The model under review builds one solid part; all positions refer to its coordinate system, in mm. A direction names the side the tool comes from. Round coordinates to 2 decimals unless told otherwise and drop trailing zeros. Loops run counter-clockwise (first coordinate to the right, second up) from the corner with the lowest first, then second, coordinate; pieces in that order, holes last. Notation, with made-up numbers: (-29.5, 60) -> (0.5, 60) arc R36 cw to (0.5, 99) -> close; hole circle Ø2 at (9.25, -5). An arc over 180 degrees is marked (long way). Use a Markdown table: item, result. Add a question column.
1) Consider section B-B on x = 3.25. State how many separate pieces and enclosed holes the cut face has, plus the area to 3 significant figures.
2) For faces 1 (the flat face through (3.11, -0.98, -6.9)), 2 (the cylindrical face through (5.314, -0.083, 2.217)), 3 (the flat face through (3.106, 2.602, -6.468)), list the 3-axis set-ups (+Z, -Z, +X, -X, +Y, -Y) from which the entire face can be reached by the end or side of a thin tool; tool diameter is ignored.
3) Consider section A-A on y = 0. Give the boundary of the cut face in (x, z).
4) Insertion check: pin 1 (3.5 mm diameter, centred on y = 0, z = 4.42, fed in from +X); pin 2 (3 mm diameter, centred on x = 1, z = 7, fed in from +Y). Each pin has a flat end and moves straight along its axis. Give the tip position at first contact, or say it passes through.
5) Wall thickness on probe 1 along Z at (x, y) = (0.75, 0.25); probe 2 along Y at (x, z) = (3.5, 7.75); probe 3 along Z at (x, y) = (3.75, -0.5): over which ranges is each line inside the solid? List them lowest first.
6) Mouldability with a two-part tool opening along Y and no side actions: class faces 4 (the flat face through (3.11, -6.46, 2.6)), 5 (the cylindrical face through (3.106, 4.579, -4.564)), 6 (the flat face through (0, 0, 0)) as released by +Y, released by -Y, zero draft, split by the parting line, or undercut.
from build123d import *

# Parameters (mm, degrees)
BOSS_EXTRUDE1_DEPTH = 6.3
SKETCH2_R           = 1.1
CUT_EXTRUDE1_DEPTH  = 7.3000001
SKETCH3_R           = 2.2
CUT_EXTRUDE2_DEPTH  = 2


with BuildPart() as part:
    # Sketch1 → Boss-Extrude1 (new body)
    with BuildSketch(Plane(origin=(0, 0, 0), x_dir=(0, 0, -1), z_dir=(1, 0, 0))):
        with BuildLine():
            Line((-0.909343603, 6.400728022), (-1.05, 7.390786494))
            add(Edge.make_bspline(
                [(-0.410905417, 9.290786494), (-0.761226832, 8.915917898), (-1.03420339, 8.440297341), (-1.05, 7.390786494)],
                knots=[0, 0, 0, 0, 1, 1, 1, 1], degree=3))
            Line((-0.410905417, 9.290786494), (0.410905417, 9.290786494))
            add(Edge.make_bspline(
                [(0.410905417, 9.290786494), (0.761226832, 8.915917898), (1.03420339, 8.440297341), (1.05, 7.390786494)],
                knots=[0, 0, 0, 0, 1, 1, 1, 1], degree=3))
            Line((1.05, 7.390786494), (0.909343603, 6.400728022))
            ThreePointArc((0.909343603, 6.400728022), (1.673265127, 6.244710467), (2.41284935, 5.997864871))
            Line((2.41284935, 5.997864871), (2.786066573, 6.925608858))
            add(Edge.make_bspline(
                [(4.289538717, 8.251509833), (3.798717175, 8.102024814), (3.324502262, 7.826613608), (2.786066573, 6.925608858)],
                knots=[0, 0, 0, 0, 1, 1, 1, 1], degree=3))
            Line((4.289538717, 8.251509833), (5.001247777, 7.840604417))
            add(Edge.make_bspline(
                [(5.001247777, 7.840604417), (5.117200723, 7.340797982), (5.115795079, 6.792410217), (4.604719921, 5.875608858)],
                knots=[0, 0, 0, 0, 1, 1, 1, 1], degree=3))
            Line((4.604719921, 5.875608858), (3.987878672, 5.088521268))
            ThreePointArc((3.987878672, 5.088521268), (4.57144534, 4.57144534), (5.088521268, 3.987878672))
            Line((5.088521268, 3.987878672), (5.875608858, 4.604719921))
            add(Edge.make_bspline(
                [(7.840604417, 5.001247777), (7.340797982, 5.117200723), (6.792410217, 5.115795079), (5.875608858, 4.604719921)],
                knots=[0, 0, 0, 0, 1, 1, 1, 1], degree=3))
            Line((7.840604417, 5.001247777), (8.251509833, 4.289538717))
            add(Edge.make_bspline(
                [(8.251509833, 4.289538717), (8.102024814, 3.798717175), (7.826613608, 3.324502262), (6.925608858, 2.786066573)],
                knots=[0, 0, 0, 0, 1, 1, 1, 1], degree=3))
            Line((6.925608858, 2.786066573), (5.997864871, 2.41284935))
            ThreePointArc((5.997864871, 2.41284935), (6.244710467, 1.673265127), (6.400728022, 0.909343603))
            Line((6.400728022, 0.909343603), (7.390786494, 1.05))
            add(Edge.make_bspline(
                [(9.290786494, 0.410905417), (8.915917898, 0.761226832), (8.440297341, 1.03420339), (7.390786494, 1.05)],
                knots=[0, 0, 0, 0, 1, 1, 1, 1], degree=3))
            Line((9.290786494, 0.410905417), (9.290786494, -0.410905417))
            add(Edge.make_bspline(
                [(9.290786494, -0.410905417), (8.915917898, -0.761226832), (8.440297341, -1.03420339), (7.390786494, -1.05)],
                knots=[0, 0, 0, 0, 1, 1, 1, 1], degree=3))
            Line((7.390786494, -1.05), (6.400728022, -0.909343603))
            ThreePointArc((6.400728022, -0.909343603), (6.244710467, -1.673265127), (5.997864871, -2.41284935))
            Line((5.997864871, -2.41284935), (6.925608858, -2.786066573))
            add(Edge.make_bspline(
                [(8.251509833, -4.289538717), (8.102024814, -3.798717175), (7.826613608, -3.324502262), (6.925608858, -2.786066573)],
                knots=[0, 0, 0, 0, 1, 1, 1, 1], degree=3))
            Line((8.251509833, -4.289538717), (7.840604417, -5.001247777))
            add(Edge.make_bspline(
                [(7.840604417, -5.001247777), (7.340797982, -5.117200723), (6.792410217, -5.115795079), (5.875608858, -4.604719921)],
                knots=[0, 0, 0, 0, 1, 1, 1, 1], degree=3))
            Line((5.875608858, -4.604719921), (5.088521268, -3.987878672))
            ThreePointArc((5.088521268, -3.987878672), (4.57144534, -4.57144534), (3.987878672, -5.088521268))
            Line((3.987878672, -5.088521268), (4.604719921, -5.875608858))
            add(Edge.make_bspline(
                [(5.001247777, -7.840604417), (5.117200723, -7.340797982), (5.115795079, -6.792410217), (4.604719921, -5.875608858)],
                knots=[0, 0, 0, 0, 1, 1, 1, 1], degree=3))
            Line((5.001247777, -7.840604417), (4.289538717, -8.251509833))
            add(Edge.make_bspline(
                [(4.289538717, -8.251509833), (3.798717175, -8.102024814), (3.324502262, -7.826613608), (2.786066573, -6.925608858)],
                knots=[0, 0, 0, 0, 1, 1, 1, 1], degree=3))
            Line((2.786066573, -6.925608858), (2.41284935, -5.997864871))
            ThreePointArc((2.41284935, -5.997864871), (1.673265127, -6.244710467), (0.909343603, -6.400728022))
            Line((0.909343603, -6.400728022), (1.05, -7.390786494))
            add(Edge.make_bspline(
                [(0.410905417, -9.290786494), (0.761226832, -8.915917898), (1.03420339, -8.440297341), (1.05, -7.390786494)],
                knots=[0, 0, 0, 0, 1, 1, 1, 1], degree=3))
            Line((0.410905417, -9.290786494), (-0.410905417, -9.290786494))
            add(Edge.make_bspline(
                [(-0.410905417, -9.290786494), (-0.761226832, -8.915917898), (-1.03420339, -8.440297341), (-1.05, -7.390786494)],
                knots=[0, 0, 0, 0, 1, 1, 1, 1], degree=3))
            Line((-1.05, -7.390786494), (-0.909343603, -6.400728022))
            ThreePointArc((-0.909343603, -6.400728022), (-1.673265127, -6.244710467), (-2.41284935, -5.997864871))
            Line((-2.41284935, -5.997864871), (-2.786066573, -6.925608858))
            add(Edge.make_bspline(
                [(-4.289538717, -8.251509833), (-3.798717175, -8.102024814), (-3.324502262, -7.826613608), (-2.786066573, -6.925608858)],
                knots=[0, 0, 0, 0, 1, 1, 1, 1], degree=3))
            Line((-4.289538717, -8.251509833), (-5.001247777, -7.840604417))
            add(Edge.make_bspline(
                [(-5.001247777, -7.840604417), (-5.117200723, -7.340797982), (-5.115795079, -6.792410217), (-4.604719921, -5.875608858)],
                knots=[0, 0, 0, 0, 1, 1, 1, 1], degree=3))
            Line((-4.604719921, -5.875608858), (-3.987878672, -5.088521268))
            ThreePointArc((-3.987878672, -5.088521268), (-4.57144534, -4.57144534), (-5.088521268, -3.987878672))
            Line((-5.088521268, -3.987878672), (-5.875608858, -4.604719921))
            add(Edge.make_bspline(
                [(-7.840604417, -5.001247777), (-7.340797982, -5.117200723), (-6.792410217, -5.115795079), (-5.875608858, -4.604719921)],
                knots=[0, 0, 0, 0, 1, 1, 1, 1], degree=3))
            Line((-7.840604417, -5.001247777), (-8.251509833, -4.289538717))
            add(Edge.make_bspline(
                [(-8.251509833, -4.289538717), (-8.102024814, -3.798717175), (-7.826613608, -3.324502262), (-6.925608858, -2.786066573)],
                knots=[0, 0, 0, 0, 1, 1, 1, 1], degree=3))
            Line((-6.925608858, -2.786066573), (-5.997864871, -2.41284935))
            ThreePointArc((-5.997864871, -2.41284935), (-6.244710467, -1.673265127), (-6.400728022, -0.909343603))
            Line((-6.400728022, -0.909343603), (-7.390786494, -1.05))
            add(Edge.make_bspline(
                [(-9.290786494, -0.410905417), (-8.915917898, -0.761226832), (-8.440297341, -1.03420339), (-7.390786494, -1.05)],
                knots=[0, 0, 0, 0, 1, 1, 1, 1], degree=3))
            Line((-9.290786494, -0.410905417), (-9.290786494, 0.410905417))
            add(Edge.make_bspline(
                [(-9.290786494, 0.410905417), (-8.915917898, 0.761226832), (-8.440297341, 1.03420339), (-7.390786494, 1.05)],
                knots=[0, 0, 0, 0, 1, 1, 1, 1], degree=3))
            Line((-7.390786494, 1.05), (-6.400728022, 0.909343603))
            ThreePointArc((-6.400728022, 0.909343603), (-6.244710467, 1.673265127), (-5.997864871, 2.41284935))
            Line((-5.997864871, 2.41284935), (-6.925608858, 2.786066573))
            add(Edge.make_bspline(
                [(-8.251509833, 4.289538717), (-8.102024814, 3.798717175), (-7.826613608, 3.324502262), (-6.925608858, 2.786066573)],
                knots=[0, 0, 0, 0, 1, 1, 1, 1], degree=3))
            Line((-8.251509833, 4.289538717), (-7.840604417, 5.001247777))
            add(Edge.make_bspline(
                [(-7.840604417, 5.001247777), (-7.340797982, 5.117200723), (-6.792410217, 5.115795079), (-5.875608858, 4.604719921)],
                knots=[0, 0, 0, 0, 1, 1, 1, 1], degree=3))
            Line((-5.875608858, 4.604719921), (-5.088521268, 3.987878672))
            ThreePointArc((-5.088521268, 3.987878672), (-4.57144534, 4.57144534), (-3.987878672, 5.088521268))
            Line((-3.987878672, 5.088521268), (-4.604719921, 5.875608858))
            add(Edge.make_bspline(
                [(-5.001247777, 7.840604417), (-5.117200723, 7.340797982), (-5.115795079, 6.792410217), (-4.604719921, 5.875608858)],
                knots=[0, 0, 0, 0, 1, 1, 1, 1], degree=3))
            Line((-5.001247777, 7.840604417), (-4.289538717, 8.251509833))
            add(Edge.make_bspline(
                [(-4.289538717, 8.251509833), (-3.798717175, 8.102024814), (-3.324502262, 7.826613608), (-2.786066573, 6.925608858)],
                knots=[0, 0, 0, 0, 1, 1, 1, 1], degree=3))
            Line((-2.786066573, 6.925608858), (-2.41284935, 5.997864871))
            ThreePointArc((-2.41284935, 5.997864871), (-1.673265127, 6.244710467), (-0.909343603, 6.400728022))
        make_face()
    extrude(amount=BOSS_EXTRUDE1_DEPTH)

    # Sketch2 → Cut-Extrude1 (cut, through all)
    with BuildSketch(Plane(origin=(6.3, 0, 0), x_dir=(0, 0, -1), z_dir=(1, 0, 0))):
        with Locations((4.415267157, 0)):
            Circle(SKETCH2_R)
        with Locations((-4.415267157, 0)):
            Circle(SKETCH2_R)
    extrude(amount=-CUT_EXTRUDE1_DEPTH, mode=Mode.SUBTRACT)

    # Sketch3 → Cut-Extrude2 (cut)
    with BuildSketch(Plane(origin=(6.3, 0, 0), x_dir=(0, 0, -1), z_dir=(1, 0, 0))):
        with Locations((-4.415267157, 0)):
            Circle(SKETCH3_R)
        with Locations((4.415267157, 0)):
            Circle(SKETCH3_R)
    extrude(amount=-CUT_EXTRUDE2_DEPTH, mode=Mode.SUBTRACT)


solid = part.part
Result set:
| question | item | result |
|---|---|---|
| 1 | separate pieces | 1 |
| 1 | enclosed holes | 2 |
| 1 | area | 186 mm2 |
| 2 | face 1 | +X, -X |
| 2 | face 2 | +X |
| 2 | face 3 | -Z, +X, -X |
| 3 | outline | (0, -9.29) -> (6.3, -9.29) -> (6.3, -6.62) -> (4.3, -6.62) -> (4.3, -5.52) -> (0, -5.52) -> close; (0, -3.32) -> (4.3, -3.32) -> (4.3, -2.22) -> (6.3, -2.22) -> (6.3, 2.22) -> (4.3, 2.22) -> (4.3, 3.32) -> (0, 3.32) -> close; (0, 5.52) -> (4.3, 5.52) -> (4.3, 6.62) -> (6.3, 6.62) -> (6.3, 9.29) -> (0, 9.29) -> close |
| 4 | pin 1 | x = 4.3 |
| 4 | pin 2 | y = 5.06 |
| 5 | probe 1 | -9.29 to -5.49, -3.34 to 3.34, 5.49 to 9.29 |
| 5 | probe 2 | -5.02 to -3.42, -1.03 to 1.03, 3.42 to 5.02 |
| 5 | probe 3 | -9.19 to -5.4, -3.44 to 3.44, 5.4 to 9.19 |
| 6 | face 4 | released by -Y |
| 6 | face 5 | undercut |
| 6 | face 6 | zero draft |
